Check sheet for the modelled part. Datum: model origin and axes. Units: mm. Give positions to 0.01 mm unless a question says otherwise; leave off trailing zeros. Write each loop counter-clockwise with the first axis right and the second up, starting at its lowest first coordinate (ties: lowest second). Pieces come first, ordered by that corner, then holes. Notation, with made-up numbers: (86.25, -35.5) -> (143.25, -35.5) arc R15 ccw to (143.25, -9.5) -> close; hole circle Ø10 at (69.5, -8.5). An arc over 180 degrees is marked (long way). Use a Markdown table: item, result. Add a question column.
1. Cross-section at B-B (z = 2.5). Enter the section's corners in (x, y), then the cut area to 3 significant figures.
2. Gauge pin test, flat end, axial feed: P1, Ø0.9, axis at x = -13.86, y = 92, coming from the +Z side. Record the tip position at first contact, or that the pin passes through.
3. Cross-section at C-C (x = 4). Enter the section's corners in (y, z).
4. Cross-section at A-A (y = -84). Enter the section's corners in (x, z), then the cut area to 3 significant figures.
5. Scan lines: probe 1 along Y at (x, z) = (0, 5.75); probe 2 along X at (y, z) = (92, 2.5); probe 3 along X at (y, z) = (68, 6.5). Record each from-to range of solid material in increasing order. Write a range as [from, to].
6. Release check for a two-part mould opening along X. For faces 1 (the cylindrical face through (0, -66, 5)), 2 (the cylindrical face through (-14.117, -90.017, 5.07)), 3 (the flat face through (20.5, -1, 5)), 4 (the flat face through (0, 1, 10)) record: released by +X, released by -X, zero draft, split by the parting line, or undercut.
from build123d import *

# Parameters (mm, degrees)
F0_W     = 41
F0_H     = 200
F1_DEPTH = 10
F2_R     = 2
F2_R_2   = 0.75
F2_R_3   = 10.5
F3_DEPTH = 25
F4_DEPTH = 25


with BuildPart() as f1:
    # F0 (on Top) → F1 (new body)
    with BuildSketch(Plane.XY):
        Rectangle(F0_W, F0_H)
    extrude(amount=F1_DEPTH)

    # F2 (on face) → F3 (cut)
    with BuildSketch(Plane.XY.offset(10)):
        with Locations((0, -68)):
            Circle(F2_R)
        with Locations((-13.856406, -92)):
            Circle(F2_R)
        with Locations((13.856406, -92)):
            Circle(F2_R)
        with Locations((0, 68)):
            Circle(F2_R_2)
        with Locations((-13.856406, 92)):
            Circle(F2_R_2)
        with Locations((13.856406, 92)):
            Circle(F2_R_2)
        with Locations((0, -84)):
            Circle(F2_R_3)
    extrude(amount=-F3_DEPTH, mode=Mode.SUBTRACT)

    # F2 (on face) → F4 (cut)
    with BuildSketch(Plane.XY.offset(10)):
        with Locations((0, -68)):
            Circle(F2_R)
        with Locations((-13.856406, -92)):
            Circle(F2_R)
        with Locations((13.856406, -92)):
            Circle(F2_R)
        with Locations((0, 68)):
            Circle(F2_R_2)
        with Locations((-13.856406, 92)):
            Circle(F2_R_2)
        with Locations((13.856406, 92)):
            Circle(F2_R_2)
        with Locations((0, -84)):
            Circle(F2_R_3)
    extrude(amount=-F4_DEPTH, mode=Mode.SUBTRACT)


solid = f1.part
Worked answers:
| question | item | result |
|---|---|---|
| 1 | outline | (-20.5, -100) -> (20.5, -100) -> (20.5, 100) -> (-20.5, 100) -> close; hole circle Ø4 at (-13.86, -92); hole circle Ø1.5 at (-13.86, 92); hole circle Ø21 at (0, -84); hole circle Ø4 at (0, -68); hole circle Ø1.5 at (0, 68); hole circle Ø4 at (13.86, -92); hole circle Ø1.5 at (13.86, 92) |
| 1 | area | 7,810 mm² |
| 2 | P1 | passes through |
| 3 | outline | (-100, 0) -> (-93.71, 0) -> (-93.71, 10) -> (-100, 10) -> close; (-74.29, 0) -> (100, 0) -> (100, 10) -> (-74.29, 10) -> close |
| 4 | outline | (-20.5, 0) -> (-10.5, 0) -> (-10.5, 10) -> (-20.5, 10) -> close; (10.5, 0) -> (20.5, 0) -> (20.5, 10) -> (10.5, 10) -> close |
| 4 | area | 200 mm² |
| 5 | probe 1 | y = [-100, -94.5], [-73.5, -70], [-66, 67.25], [68.75, 100] |
| 5 | probe 2 | x = [-20.5, -14.61], [-13.11, 13.11], [14.61, 20.5] |
| 5 | probe 3 | x = [-20.5, -0.75], [0.75, 20.5] |
| 6 | face 1 | undercut |
| 6 | face 2 | undercut |
| 6 | face 3 | released by +X |
| 6 | face 4 | zero draft |
